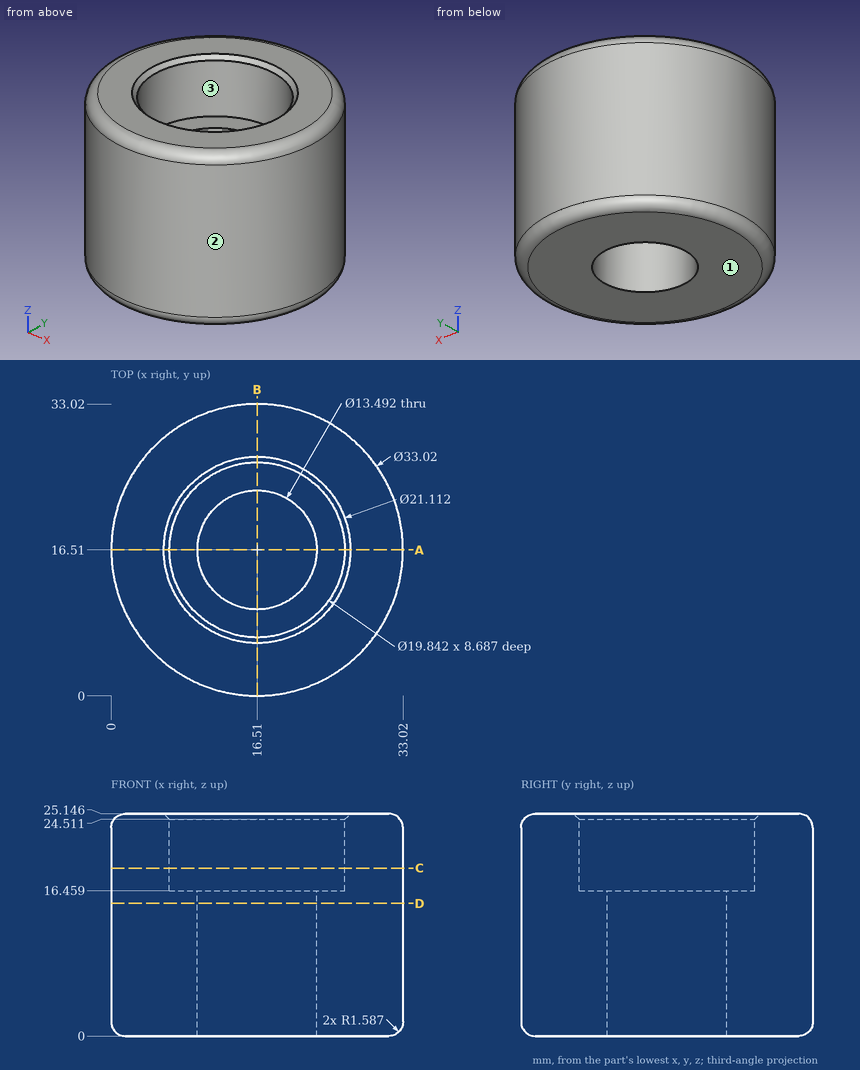
Study the drawing (mm; zero at the part's minimum x, y, z) and answer. Give positions to 0.01 mm unless a question says otherwise; leave off trailing zeros. Loops run counter-clockwise (first coordinate to the right, second up) from the corner with the lowest first, then second, coordinate; pieces in that order, holes last. Notation, with made-up numbers: (-30.5, 7) - (14.5, 7) arc R20 cw to (14.5, 34) - close; hole circle Ø3 at (-22, 35). An arc over 180 degrees is marked (long way). Return JSON: item names as keys, results as strings. Group by question number.
1. Find section C-C (z = 19). Write down the section's boundary in (x, y), then the cut area to 3 significant figures.
2. Determine the mould class of the marked faces 1, 2 and 3 for opening direction X: pulls with the +X half, pulls with the -X half, needs draft (parallel to the pull), parting line crosses it, or undercut.
3. Find section D-D (z = 15). Write down the section's boundary in (x, y).
4. Straight lines are drawn through the part: line 1 (Z direction, x = 19.5, y = 25.5); line 2 (X direction, y = 11.5, z = 10.75) (1 decimal); line 3 (Z direction, x = 31, y = 12.5) (1 decimal). For each, find the intervals that lie inside material, in ascending order. Write a range as [from, to].
5. Given pin 1 Ø4 at (x, y) = (8.5, 7.5) entering from -Z; pin 2 Ø12 at (x, z) = (3.5, 7.5) entering from +Y; pin 3 Ø1 at (x, z) = (14.5, 19.5) entering from -Y; pin 4 Ø15.5 at (x, y) = (16.51, 16.51) entering from +Z, each flat-ended and moving along its own axis, determine where each tip first touches the part or whether it passes through.
6. Find section A-A (y = 16.51). Write down the section's boundary in (x, z) (1 decimal).
Verdict:
{
 "1": {"outline": "circle Ø33.02 at (16.51, 16.51); hole circle Ø19.84 at (16.51, 16.51)", "area": "547 mm^2"},
 "2": {"face 1": "needs draft", "face 2": "parting line crosses it", "face 3": "undercut"},
 "3": {"outline": "circle Ø33.02 at (16.51, 16.51); hole circle Ø13.49 at (16.51, 16.51)"},
 "4": {"line 1": "z = [0, 16.46]", "line 2": "x = [0.8, 12], [21, 32.2]", "line 3": "z = [0, 25.1]"},
 "5": {"pin 1": "stops at z = 0", "pin 2": "stops at y = 31.46", "pin 3": "stops at y = 0.07", "pin 4": "stops at z = 16.46"},
 "6": {"outline": "(0, 1.6) arc R1.6 ccw to (1.6, 0) - (9.8, 0) - (9.8, 16.5) - (6.6, 16.5) - (6.6, 24.5) - (6, 25.1) - (1.6, 25.1) arc R1.6 ccw to (0, 23.6) - close; (23.3, 0) - (31.4, 0) arc R1.6 ccw to (33, 1.6) - (33, 23.6) arc R1.6 ccw to (31.4, 25.1) - (27.1, 25.1) - (26.4, 24.5) - (26.4, 16.5) - (23.3, 16.5) - close"}
}
